from build123d import *

# Parameters (mm, degrees)
SKETCH1_R           = 7.5
BOSS_EXTRUDE5_DEPTH = 7.5
SKETCH7_R           = 3.25
SKETCH7_R_2         = 2.5
BOSS_EXTRUDE6_DEPTH = 0.5
SKETCH8_R           = 2
BOSS_EXTRUDE7_DEPTH = 8
CUT_EXTRUDE2_START  = -3
CUT_EXTRUDE2_DEPTH  = 3
SKETCH10_W          = 20
SKETCH10_H          = 10
BOSS_EXTRUDE8_DEPTH = 7.5
FILLET2_R           = 2


with BuildPart() as part:
    # Sketch1 → Boss-Extrude5 (new, symmetric)
    with BuildSketch(Plane.XY):
        Circle(SKETCH1_R)
    extrude(amount=BOSS_EXTRUDE5_DEPTH, both=True)

    # Sketch7 → Boss-Extrude6 (add)
    with BuildSketch(Plane.XY.offset(7.5)):
        Circle(SKETCH7_R)
        Circle(SKETCH7_R_2, mode=Mode.SUBTRACT)
    extrude(amount=BOSS_EXTRUDE6_DEPTH)

    # Sketch8 → Boss-Extrude7 (add)
    with BuildSketch(Plane.XY.offset(7.5)):
        Circle(SKETCH8_R)
    extrude(amount=BOSS_EXTRUDE7_DEPTH)

    # Sketch9 → Cut-Extrude2 (cut)
    with BuildSketch(Plane.XY.offset(15.5).offset(CUT_EXTRUDE2_START)):
        with BuildLine():
            Line((-2, 0), (2, 0))
            ThreePointArc((2, 0), (0, -2), (-2, 0))
        make_face()
    extrude(amount=CUT_EXTRUDE2_DEPTH, mode=Mode.SUBTRACT)

    # Sketch10 → Boss-Extrude8 (add)
    with BuildSketch(Plane(origin=(0, 0, 0), x_dir=(1, 0, 0), z_dir=(0, 1, 0))):
        Rectangle(SKETCH10_W, SKETCH10_H)
    extrude(amount=-BOSS_EXTRUDE8_DEPTH)

    # Fillet2
    fillet2_edges = [part.edges().sort_by_distance(p)[0] for p in [
        (-7.5, 0, -7.5),
        (-7.5, 0, 7.5),
    ]]
    fillet(fillet2_edges, radius=FILLET2_R)


solid = part.part
Work out the finished part from the listing and answer in its coordinate system (mm). A direction names the side the tool comes from. Give positions to 0.01 mm unless a question says otherwise; leave off trailing zeros. Order: outer loops, then holes, each group sorted by start corner. A loop starts at its lowest first (then second) coordinate and runs counter-clockwise, first axis right, second up. Notation, with made-up numbers: M 75,84.25 L 91,84.25 A18 ccw 91,112.25 Z; hole C 2.25,8 d7. An arc over 180 degrees is marked long. Return JSON: item names as keys, results as strings.
Q1. Find section C-C, the plane z = 6. Write down the section's boundary in (x, y), and give its area (3 significant figures).
Answer below:
{"outline": "C 0,0 d14.87", "area": "174 mm^2"}
Q2. Find section A-A, the plane z = 1. Write down the section's boundary in (x, y), and give its area (3 significant figures).
Answer below:
{"outline": "M -10,-7.5 L 10,-7.5 L 10,0 L 7.5,0 A7.5 ccw -7.5,0 L -10,0 Z", "area": "238 mm^2"}
Q3. Each of these flat-tipped pins is pushed along its axis until it touches: pin 1 (2 mm diameter, centred on x = 4.5, y = -4.5, fed in from +Z); pin 2 (8.5 mm diameter, centred on x = -4, y = -5.5, fed in from +Z); pin 3 (4 mm diameter, centred on x = 7.5, y = -6, fed in from +Z); pin 4 (1.5 mm diameter, centred on x = -1, y = -0.5, fed in from +Z). Where does it stop, or does it pass through?
Answer below:
{"pin 1": "stops at z = 7.5", "pin 2": "stops at z = 8", "pin 3": "stops at z = 5", "pin 4": "stops at z = 15.5"}
Q4. Which of the six approach directions +Z, -Z, +X, -X, +Y, -Y give full straight-line access (tool end or side, diameter ignored) to faces 5 (the face through (0, 0, 14)), 6 (the face through (-9, 0, 0)), 7 (the face through (9, 0, 0)), 8 (the face through (0, 2, 11))?
Answer below:
{"face 5": "+Z, +X, -X, -Y", "face 6": "+Z, -Z, -X, +Y", "face 7": "+Z, -Z, +X, +Y", "face 8": "+Z"}
Q5. Find section B-B, the plane z = 13. Write down the section's boundary in (x, y), and give its area (3 significant figures).
Answer below:
{"outline": "M -2,0 L 2,0 A2 ccw Z", "area": "6.28 mm^2"}
Q6. The mould has two halves that part along X. Classify faces 1 (the face through (-1, 2, 7.5)), 2 (the face through (-0.54, -2.44, 7.75)), 3 (the face through (0, -1, 12.5)), 4 (the face through (-0.976, 7.436, 0.077)): pulls with the +X half, pulls with the -X half, needs draft (parallel to the pull), parting line crosses it, or undercut.
Answer below:
{"face 1": "undercut", "face 2": "undercut", "face 3": "needs draft", "face 4": "parting line crosses it"}
Q7. Find the intervals of material crossed by line 1 along Y through (x, z) = (0, 7.8); line 2 along Z through (x, y) = (5.25, -0.5); line 3 along Z through (x, y) = (0.5, -1.5), in increasing order. Write a range as [from, to].
Answer below:
{"line 1": "y = [-3.25, -2.5], [-2, 2], [2.5, 3.25]", "line 2": "z = [-7.5, 7.5]", "line 3": "z = [-7.5, 12.5]"}
